from build123d import *

# Parameters (mm, degrees)
SKETCH1_W   = 14
SKETCH1_H   = 5.5
SKETCH1_W_2 = 12.5
SKETCH1_H_2 = 6.75


with BuildPart() as part:
    # Sketch1 → Revolve2 (revolve)
    with BuildSketch(Plane(origin=(0, 0, 0), x_dir=(0, 0, -1), z_dir=(1, 0, 0)), mode=Mode.PRIVATE) as revolve2_sk:
        with Locations((7, 2.75)):
            Rectangle(SKETCH1_W, SKETCH1_H)
        Polygon((14, 5.5), (14, 0), (25, 0), (25, 7), (14, 7), align=None)
        Polygon((25, 7), (25, 0), (52, 0), (52, 8.5), (52, 10.25), (25, 10.25), align=None)
        Polygon((52, 8.5), (52, 0), (59.5, 0), (59.5, 6.75), (59.5, 8.5), align=None)
        with Locations((65.75, 3.375)):
            Rectangle(SKETCH1_W_2, SKETCH1_H_2)
    revolve(revolve2_sk.sketch.rotate(Axis((0, 0, -25), (0, 0, -1)), 90), axis=Axis((0, 0, -25), (0, 0, -1)))


solid = part.part
The listing builds one solid part. Answer for the finished solid, in the listing's coordinates (mm). A direction names the side the tool comes from. Coordinates: 2 decimals unless noted, no trailing zeros. Loops run counter-clockwise (first coordinate to the right, second up) from the corner with the lowest first, then second, coordinate; pieces in that order, holes last. Notation, with made-up numbers: (15, -14) -> (42, -14) arc R15 ccw to (42, -8) -> close; hole circle Ø7 at (-29, 84). An arc over 180 degrees is marked (long way). Answer in a Markdown table with one row per item. Add a question column.
1. For faces 1 (the flat face through (0, 0, -72)), 2 (the cylindrical face through (-1.19, 5.37, -7.1)), 3 (the flat face through (-1, -7, -59.5)), determine the directions among +Z, -Z, +X, -X, +Y, -Y from which every point of the face is accessible in a straight line to the end or side of a thin tool.
2. The part is cut by section A-A, the plane y = 0. Write down the section's boundary in (x, z).
3. Flat-ended cylindrical pins translate along their axes: P1, Ø10, axis at y = 3, z = -18, coming from the +X side; P2, Ø1.5, axis at x = 7, y = 3.5, coming from the -Z side; P3, Ø1.5, axis at x = -5, z = -9, coming from the +Y side. Find the tip coordinate at first contact, or state that the pin passes through.
4. The part is cut by section D-D, the plane z = -58. Write down the section's boundary in (x, y), then the cut area to 3 significant figures.
5. The part is cut by section C-C, the plane z = -23.5. Write down the section's boundary in (x, y).
6. Consider line 1 (X direction, y = -0.25, z = -54); line 2 (Z direction, x = -4.5, y = 7); line 3 (Z direction, x = -9, y = -1.5). Determine where each line is inside the solid, lowest interval first. Write a range as [from, to].
Answer below:
| question | item | result |
|---|---|---|
| 1 | face 1 | -Z, +X, -X, +Y, -Y |
| 1 | face 2 | +Z |
| 1 | face 3 | -Z |
| 2 | outline | (-10.25, -52) -> (-8.5, -52) -> (-8.5, -59.5) -> (-6.75, -59.5) -> (-6.75, -72) -> (6.75, -72) -> (6.75, -59.5) -> (8.5, -59.5) -> (8.5, -52) -> (10.25, -52) -> (10.25, -25) -> (7, -25) -> (7, -14) -> (5.5, -14) -> (5.5, 0) -> (-5.5, 0) -> (-5.5, -14) -> (-7, -14) -> (-7, -25) -> (-10.25, -25) -> close |
| 3 | P1 | x = 7 |
| 3 | P2 | z = -59.5 |
| 3 | P3 | y = 3.49 |
| 4 | outline | circle Ø17 at (0, 0) |
| 4 | area | 227 mm2 |
| 5 | outline | circle Ø14 at (0, 0) |
| 6 | line 1 | [-8.5, 8.5] |
| 6 | line 2 | [-59.5, -25] |
| 6 | line 3 | [-52, -25] |
